from build123d import *

# Parameters (mm, degrees)
FILLET1_R = 3.175


with BuildPart() as part:
    # Sketch1 → Revolve1 (revolve)
    with BuildSketch(Plane.XY, mode=Mode.PRIVATE) as revolve1_sk:
        Polygon((35.586256664, 107.95), (48.286256664, 107.95), (48.286256664, 12.7), (60.986256664, 12.7), (60.986256664, 0), (35.586256664, 0), align=None)
    revolve(revolve1_sk.sketch.rotate(Axis((0, 107.95, 0), (0, -1, 0)), 90), axis=Axis((0, 107.95, 0), (0, -1, 0)))

    # Fillet1
    fillet1_edges = [part.edges().sort_by_distance(p)[0] for p in [
        (0, 107.95, -35.586256664),
        (0, 107.95, -48.286256664),
        (0, 12.7, -48.286256664),
    ]]
    fillet(fillet1_edges, radius=FILLET1_R)


solid = part.part
Could you check a few things on this model? Use its own coordinates, in mm. A direction names the side the tool comes from. Give positions to 0.01 mm unless a question says otherwise; leave off trailing zeros. Order: outer loops, then holes, each group sorted by start corner. A loop starts at its lowest first (then second) coordinate and runs counter-clockwise, first axis right, second up.
Item 1: For faces 4 (the face through (13, 12.7, 50)), 5 (the face through (-34, 107.95, -20)), which set-ups out of +Z, -Z, +X, -X, +Y, -Y let a thin tool reach every point of the face, with its end or its side?
Item 2: If we mould it in two halves opening along Z, with no side actions, what happens to faces 1 (the face through (21.654, 53.121, -28.24)), 2 (the face through (26, 0, 26)), 3 (the face through (-18.32, 6.26, 58.17))? For each: pulls with the +Z half, pulls with the -Z half, needs draft (parallel to the pull), parting line crosses it, or undercut.
Item 3: I need wall thicknesses on line 1 (X direction, y = 62, z = 0); line 2 (Y direction, x = -38, z = 47.5); line 3 (Z direction, x = 5, y = 94.5). Which ranges of each line are inside material? Lowest first, please.
Item 4: If we section it at A-A, the plane x = 0: Write out the boundary of the cut face in (y, z) (3 decimals).
Item 5: If we section it at B-B, the plane z = 0: Write out the boundary of the cut face in (x, y) (3 decimals).
Item 6: If we section it at D-D, the plane y = 57.5: Write out the boundary of the cut face in (x, z).
Item 7: If we section it at C-C, the plane y = 9.5: Write out the boundary of the cut face in (x, z).
Item 8: I'm going to push flat-ended pins straight in: pin 1 (4 mm diameter, centred on y = 81, z = 10, fed in from -X); pin 2 (5 mm diameter, centred on x = 6.5, y = 67.5, fed in from +Z); pin 3 (3 mm diameter, centred on x = -20.5, y = 37.5, fed in from -Z). Where does each tip first touch, or does it pass through?
Values:
1. face 4: +Y
1. face 5: +Z, -Z, +X, -X, +Y
2. face 1: undercut
2. face 2: needs draft
2. face 3: parting line crosses it
3. line 1: x = -48.29 to -35.59, 35.59 to 48.29
3. line 2: y = 0 to 12.7
3. line 3: z = -48.03 to -35.23, 35.23 to 48.03
4. outline: (0, -60.986) - (12.7, -60.986) - (12.7, -51.461) arc R3.175 cw to (15.875, -48.286) - (104.775, -48.286) arc R3.175 ccw to (107.95, -45.111) - (107.95, -38.761) arc R3.175 ccw to (104.775, -35.586) - (0, -35.586) - close; (0, 35.586) - (104.775, 35.586) arc R3.175 ccw to (107.95, 38.761) - (107.95, 45.111) arc R3.175 ccw to (104.775, 48.286) - (15.875, 48.286) arc R3.175 cw to (12.7, 51.461) - (12.7, 60.986) - (0, 60.986) - close
5. outline: (-60.986, 0) - (-35.586, 0) - (-35.586, 104.775) arc R3.175 ccw to (-38.761, 107.95) - (-45.111, 107.95) arc R3.175 ccw to (-48.286, 104.775) - (-48.286, 15.875) arc R3.175 cw to (-51.461, 12.7) - (-60.986, 12.7) - close; (35.586, 0) - (60.986, 0) - (60.986, 12.7) - (51.461, 12.7) arc R3.175 cw to (48.286, 15.875) - (48.286, 104.775) arc R3.175 ccw to (45.111, 107.95) - (38.761, 107.95) arc R3.175 ccw to (35.586, 104.775) - close
6. outline: circle Ø96.57 at (0, 0); hole circle Ø71.17 at (0, 0)
7. outline: circle Ø121.97 at (0, 0); hole circle Ø71.17 at (0, 0)
8. pin 1: stops at x = -47.62
8. pin 2: stops at z = 48.12
8. pin 3: stops at z = -44.39
